For this review, take the finished solid that the model builds, in its own axes (mm). Face numbers are marked on the shaded views. A direction names the side the tool comes from. Give positions to 0.01 mm unless a question says otherwise; leave off trailing zeros. Loops run counter-clockwise (first coordinate to the right, second up) from the corner with the lowest first, then second, coordinate; pieces in that order, holes last.
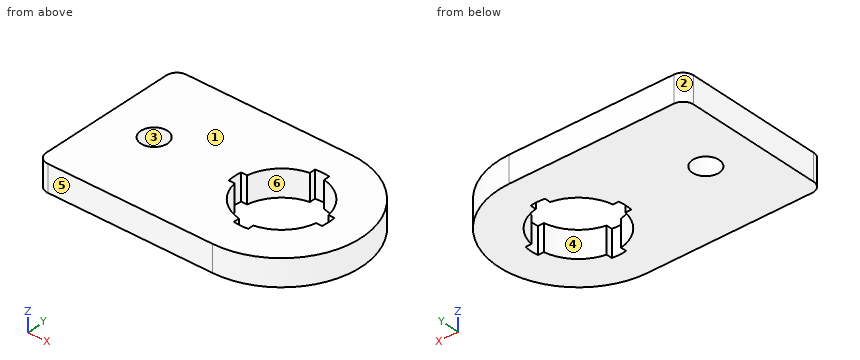
```python
from build123d import *

# Parameters (mm, degrees)
SKETCH_R  = 2.5
PAD_DEPTH = 5


with BuildPart() as part:
    # Sketch → Pad (new body)
    with BuildSketch(Plane.XY):
        with BuildLine():
            Line((-7, 15), (24, 15))
            ThreePointArc((24, -15), (39, 0), (24, 15))
            Line((-7, -15), (24, -15))
            ThreePointArc((-9, -13), (-8.414214, -14.414214), (-7, -15))
            Line((-9, 13), (-9, -13))
            ThreePointArc((-7, 15), (-8.414214, 14.414214), (-9, 13))
        make_face()
        Circle(SKETCH_R, mode=Mode.SUBTRACT)
        with BuildLine():
            ThreePointArc((16.317715, -1.35), (18.484567, -5.515433), (22.65, -7.682285))
            Line((22.65, -7.682285), (22.65, -8.797017))
            ThreePointArc((22.65, -8.797017), (24, -8.9), (25.35, -8.797017))
            Line((25.35, -7.682285), (25.35, -8.797017))
            ThreePointArc((25.35, -7.682285), (29.515433, -5.515433), (31.682285, -1.35))
            Line((31.682285, -1.35), (32.797017, -1.35))
            ThreePointArc((32.797017, -1.35), (32.9, 0), (32.797017, 1.35))
            Line((31.682285, 1.35), (32.797017, 1.35))
            ThreePointArc((31.682285, 1.35), (29.515433, 5.515433), (25.35, 7.682285))
            Line((25.35, 8.797017), (25.35, 7.682285))
            ThreePointArc((25.35, 8.797017), (24, 8.9), (22.65, 8.797017))
            Line((22.65, 8.797017), (22.65, 7.682285))
            ThreePointArc((22.65, 7.682285), (18.484567, 5.515433), (16.317715, 1.35))
            Line((15.202983, 1.35), (16.317715, 1.35))
            ThreePointArc((15.202983, 1.35), (15.1, 0), (15.202983, -1.35))
            Line((15.202983, -1.35), (16.317715, -1.35))
        make_face(mode=Mode.SUBTRACT)
    extrude(amount=PAD_DEPTH)


solid = part.part
```
Q1. Consider section D-D on x = 35. Give the boundary of the cut face in (y, z), plus the area to 3 significant figures.
Answers:
outline: (-10.2, 0) - (10.2, 0) - (10.2, 5) - (-10.2, 5) - close
area: 102 mm2
Q2. Consider section A-A on x = 0. Give the boundary of the cut face in (y, z).
Answers:
outline: (-15, 0) - (-2.5, 0) - (-2.5, 5) - (-15, 5) - close; (2.5, 0) - (15, 0) - (15, 5) - (2.5, 5) - close
Q3. Consider section B-B on y = 0. Give the boundary of the cut face in (x, z).
Answers:
outline: (-9, 0) - (-2.5, 0) - (-2.5, 5) - (-9, 5) - close; (2.5, 0) - (15.1, 0) - (15.1, 5) - (2.5, 5) - close; (32.9, 0) - (39, 0) - (39, 5) - (32.9, 5) - close
Q4. For probe 1 along Y at (x, z) = (0, 3.5); probe 2 along X at (y, z) = (-2, 4.15); probe 3 along X at (y, z) = (-4.5, 2.5), list the stretches that pass through material, from the lowest coordinate up.
Answers:
probe 1: y = -15 to -2.5, 2.5 to 15
probe 2: x = -9 to -1.5, 1.5 to 16.46, 31.54 to 38.87
probe 3: x = -9 to 17.63, 30.37 to 38.31
Q5. Consider section C-C on z = 1.9. Give the boundary of the cut face in (x, y).
Answers:
outline: (-9, -13) arc R2 ccw to (-7, -15) - (24, -15) arc R15 ccw to (24, 15) - (-7, 15) arc R2 ccw to (-9, 13) - close; hole circle Ø5 at (0, 0); hole (15.2, -1.35) - (16.32, -1.35) arc R7.8 ccw to (22.65, -7.68) - (22.65, -8.8) arc R8.9 ccw to (25.35, -8.8) - (25.35, -7.68) arc R7.8 ccw to (31.68, -1.35) - (32.8, -1.35) arc R8.9 ccw to (32.8, 1.35) - (31.68, 1.35) arc R7.8 ccw to (25.35, 7.68) - (25.35, 8.8) arc R8.9 ccw to (22.65, 8.8) - (22.65, 7.68) arc R7.8 ccw to (16.32, 1.35) - (15.2, 1.35) arc R8.9 ccw to start
Q6. Machinability: for the marked faces 5 and 6, which of the approach directions +Z, -Z, +X, -X, +Y, -Y give a long, thin tool a straight path to every point of the face, cutting with its end or side? Answer none if there is none.
Answers:
face 5: +Z, -Z, +X, -X, -Y
face 6: +Z, -Z
Q7. Mouldability with a two-part tool opening along X and no side actions: class the marked faces 1, 2, 3 and 4 as +X half, -X half, draft (parallel to the pull), parting line (faces both ways), or undercut.
Answers:
face 1: draft
face 2: -X half
face 3: undercut
face 4: undercut
Q8. For pin 1 Ø0.6 at (x, z) = (32, 2) entering from -Y; pin 2 Ø1.2 at (y, z) = (8, 1.5) entering from +X; pin 3 Ø4 at (x, y) = (0, 0) entering from -Z; pin 4 Ø1.2 at (x, z) = (32, 2) entering from +Y, all flat-tipped, find the tip position at first contact; note any pin that passes through.
Answers:
pin 1: stops at y = -12.87
pin 2: stops at x = 37.05
pin 3: passes through
pin 4: stops at y = 13.05
